```python
from build123d import *

# Parameters (mm, degrees)
F1_DEPTH = 30
F2_R     = 5.1
F3_DEPTH = 50.0010000522
F4_R     = 14.99999
F5_R     = 3


# Not quite as in the source:
# - a fillet or chamfer is up to 0.001 mm smaller than in the source, because OpenCascade refuses the exact size


with BuildPart() as f1:
    # F0 (on Front) → F1 (new body)
    with BuildSketch(Plane.XZ):
        Polygon((-3.0000000261, 0), (0, 0), (0, 37), (44, 37), (44, 0), (47.0000000261, 0), (47.0000000261, 40.0000000261), (-3.0000000261, 40.0000000261), align=None)
    extrude(amount=F1_DEPTH)

    # F2 (on face) → F3 (cut, through all)
    with BuildSketch(Plane(origin=(-3.0000000261, 0, 0), x_dir=(0, -1, 0), z_dir=(-1, 0, 0))):
        with Locations((15, 15.0000000261)):
            Circle(F2_R)
    extrude(amount=-F3_DEPTH, mode=Mode.SUBTRACT)

    # F4 (radius 15 in the source; OpenCascade refuses exactly that, so slightly less here)
    f4_edges = [f1.edges().sort_by_distance(p)[0] for p in [
        (45.5, 0, 0),
        (45.5, -30, 0),
        (-1.5, -30, 0),
        (-1.5, 0, 0),
    ]]
    fillet(f4_edges, radius=F4_R)

    # F5
    f5_edges = [f1.edges().sort_by_distance(p)[0] for p in [
        (0, -15, 37),
        (44, -15, 37),
        (47, -15, 40),
        (-3, -15, 40),
    ]]
    fillet(f5_edges, radius=F5_R)


solid = f1.part
```
CAD build for the part. Positions are in the model's coordinates, mm. A direction names the side the tool comes from. Round coordinates to 2 decimals unless told otherwise and drop trailing zeros. Write each loop counter-clockwise with the first axis right and the second up, starting at its lowest first coordinate (ties: lowest second). Pieces come first, ordered by that corner, then holes. Notation, with made-up numbers: (-4.75, -29.5) - (41.25, -29.5) arc R31 ccw to (41.25, 3.5) - close; hole circle Ø8 at (53.25, 24.5). An arc over 180 degrees is marked (long way). Return JSON: item names as keys, results as strings. Group by question number.
Item 1: Band-saw the part on C-C on y = -4. List the corners of the cut face in (x, z), plus the area to 3 significant figures.
Item 2: 3-axis set-ups, long thin cutter, end or side, ignore diameter. For faces 1 (the face through (22, -30, 38)), 2 (the face through (43.1, -15.21, 36.14)): which of +Z, -Z, +X, -X, +Y, -Y reach the whole face in a straight line?
Item 3: Mould opens along X. For faces 3 (the face through (-2.14, -15.21, 39.1)), 4 (the face through (22, -15, 37)), 5 (the face through (22, 0, 38)), 6 (the face through (46.1, -15.21, 39.14)) say: +X half, -X half, draft (parallel to the pull), parting line (faces both ways), or undercut.
Item 4: Probe probe 1 along X at (y, z) = (-22, 33.5); probe 2 along Z at (x, y) = (27, -2); probe 3 along Z at (x, y) = (-1.75, -15). List the from-to ranges inside material, lowest first.
Item 5: Band-saw the part on A-A on z = 21.5. List the corners of the cut face in (x, y), plus the area to 3 significant figures.
Item 6: Flat gauge pin, fed straight in: pin 1 Ø1.5 at (x, y) = (38, -8.5) entering from -Z. Where does the tip first touch, or does it go through?
Item 7: Band-saw the part on B-B on y = -16. List the corners of the cut face in (x, z), plus the area to 3 significant figures.
Item 8: Band-saw the part on D-D on x = 18. List the corners of the cut face in (y, z).
Resolved:
{
 "1": {"outline": "(-3, 4.8) - (0, 4.8) - (0, 34) arc R3 cw to (3, 37) - (41, 37) arc R3 cw to (44, 34) - (44, 4.8) - (47, 4.8) - (47, 37) arc R3 ccw to (44, 40) - (0, 40) arc R3 ccw to (-3, 37) - close", "area": "343 mm²"},
 "2": {"face 1": "+Z, -Z, +X, -X, -Y", "face 2": "-Z, +Y, -Y"},
 "3": {"face 3": "-X half", "face 4": "undercut", "face 5": "draft", "face 6": "+X half"},
 "4": {"probe 1": "x = -3 to 0, 44 to 47", "probe 2": "z = 37 to 40", "probe 3": "z = 0 to 9.9, 20.1 to 39.44"},
 "5": {"outline": "(-3, -30) - (0, -30) - (0, 0) - (-3, 0) - close; (44, -30) - (47, -30) - (47, 0) - (44, 0) - close", "area": "180 mm²"},
 "6": {"pin 1": "stops at z = 37"},
 "7": {"outline": "(-3, 0.03) - (0, 0.03) - (0, 10) - (-3, 10) - close; (-3, 20) - (0, 20) - (0, 34) arc R3 cw to (3, 37) - (41, 37) arc R3 cw to (44, 34) - (44, 20) - (47, 20) - (47, 37) arc R3 ccw to (44, 40) - (0, 40) arc R3 ccw to (-3, 37) - close; (44, 0.03) - (47, 0.03) - (47, 10) - (44, 10) - close", "area": "312 mm²"},
 "8": {"outline": "(-30, 37) - (0, 37) - (0, 40) - (-30, 40) - close"}
}
